CAD build for the part. Positions are in the model's coordinates, mm. Face numbers are marked on the shaded views. Coordinates: 2 decimals unless noted, no trailing zeros. Loops run counter-clockwise (first coordinate to the right, second up) from the corner with the lowest first, then second, coordinate; pieces in that order, holes last. Notation, with made-up numbers: (67, 24) -> (115, 24) arc R30 ccw to (115, 58) -> close; hole circle Ø5 at (-10, 28). An arc over 180 degrees is marked (long way). Write item = value, one per line. Start each with the question number.
(1) Band-saw the part on A-A (y = 0). Write the cut outline in (x, z), and give its area (3 significant figures).
(2) Drill centre lines: line 1 (Y direction, x = 0, z = 33); line 2 (Z direction, x = -9, y = 16); line 3 (Y direction, x = -36, z = 3.4). Where is each one in solid material? Low to high. Write a range as from..to.
(3) Pull direction X, two halves, no side cores. Call the marked faces 1, 2 and 3: +X half, -X half, draft (parallel to the pull), parting line (faces both ways), or undercut.
(4) Flat gauge pins, fed straight in: P1, Ø5, axis at y = -9, z = 11, coming from the -X side; P2, Ø2, axis at y = -27.5, z = 36.5, coming from the -X side; P3, Ø12, axis at x = -16.5, z = 29.5, coming from the +Y side. Where does each tip first touch, or does it go through?
(5) Band-saw the part on B-B (x = 0). Write the cut outline in (y, z), and give its area (3 significant figures).
(6) Band-saw the part on C-C (z = 37). Write the cut outline in (x, y).
```python
from build123d import *

# Parameters (mm, degrees)
F0_R     = 46.5
F0_R_2   = 2
F1_DEPTH = 3
F2_R     = 46.5
F2_R_2   = 43
F3_DEPTH = 42
F4_SIZE  = 2.5
F5_R     = 2
F6_DEPTH = 2


with BuildPart() as f1:
    # F0 (on Top) → F1 (new body)
    with BuildSketch(Plane.XY):
        Circle(F0_R)
        with Locations((-36, 0)):
            Circle(F0_R_2, mode=Mode.SUBTRACT)
        with Locations((36, 0)):
            Circle(F0_R_2, mode=Mode.SUBTRACT)
    extrude(amount=F1_DEPTH)

    # F2 (on face) → F3 (join)
    with BuildSketch(Plane.XY.offset(3)):
        Circle(F2_R)
        Circle(F2_R_2, mode=Mode.SUBTRACT)
    extrude(amount=F3_DEPTH)

    # F4
    f4_edges = [f1.edges().sort_by_distance(p)[0] for p in [
        (-43, 0, 45),
    ]]
    chamfer(f4_edges, length=F4_SIZE)

    # F5 (on face) → F6 (join)
    with BuildSketch(Plane.XY.offset(3)):
        with BuildLine():
            Line((-30, -7.5), (-30, 7.5))
            Line((-30, 7.5), (-42.3408785927, 7.5))
            ThreePointArc((-42.3408785927, 7.5), (-43, 0), (-42.3408785927, -7.5))
            Line((-42.3408785927, -7.5), (-30, -7.5))
        make_face()
        with Locations((-36, 0)):
            Circle(F5_R, mode=Mode.SUBTRACT)
        with BuildLine():
            ThreePointArc((43, 0), (42.834902705, 3.7644535138), (42.3408785927, 7.5))
            Line((42.3408785927, 7.5), (30, 7.5))
            Line((30, 7.5), (30, -7.5))
            Line((30, -7.5), (42.3408785927, -7.5))
            ThreePointArc((42.3408785927, -7.5), (42.834902705, -3.7644535138), (43, 0))
        make_face()
        with Locations((36, 0)):
            Circle(F5_R, mode=Mode.SUBTRACT)
    extrude(amount=F6_DEPTH)


solid = f1.part
```
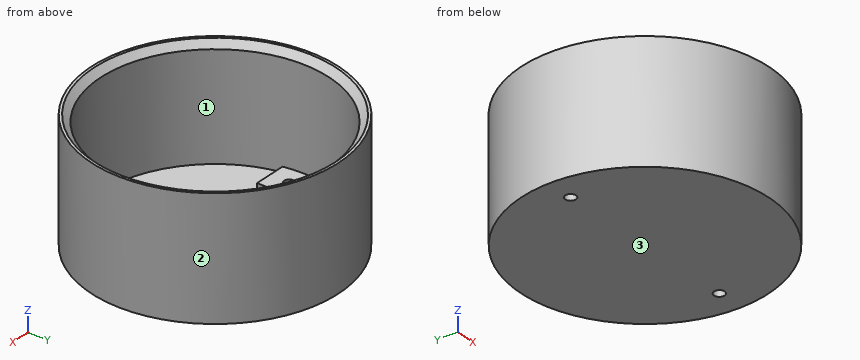
Findings below:
q1.outline = (-46.5, 0) -> (-38, 0) -> (-38, 5) -> (-43, 5) -> (-43, 42.5) -> (-45.5, 45) -> (-46.5, 45) -> close; (-34, 0) -> (34, 0) -> (34, 5) -> (30, 5) -> (30, 3) -> (-30, 3) -> (-30, 5) -> (-34, 5) -> close; (38, 0) -> (46.5, 0) -> (46.5, 45) -> (45.5, 45) -> (43, 42.5) -> (43, 5) -> (38, 5) -> close
q1.area = 579 mm²
q2.line_1 = -46.5..-43, 43..46.5
q2.line_2 = 0..3
q2.line_3 = -29.43..-23.52, -7.5..-2, 2..7.5, 23.52..29.43
q3.face_1 = undercut
q3.face_2 = parting line
q3.face_3 = draft
q4.P1 = -46.04
q4.P2 = -38.21
q4.P3 = 45.3
q5.outline = (-46.5, 0) -> (46.5, 0) -> (46.5, 45) -> (45.5, 45) -> (43, 42.5) -> (43, 3) -> (-43, 3) -> (-43, 42.5) -> (-45.5, 45) -> (-46.5, 45) -> close
q5.area = 567 mm²
q6.outline = circle Ø93 at (0, 0); hole circle Ø86 at (0, 0)
